Verification items for the finished model (mm, model axes). Face numbers are marked on the shaded views. Round coordinates to 2 decimals unless told otherwise and drop trailing zeros. Write each loop counter-clockwise with the first axis right and the second up, starting at its lowest first coordinate (ties: lowest second). Pieces come first, ordered by that corner, then holes.
from build123d import *

# Parameters (mm, degrees)
SKETCH_1_W          = 4
SKETCH_1_H          = 12
EXTRUDE_1_DEPTH     = 13
SKETCH_2_R          = 1.25
EXTRUDE_2_DEPTH     = 5
SKETCH_3_R          = 1
CUT_EXTRUDE_1_DEPTH = 22.771541057


with BuildPart() as part:
    # 草图1 → 凸台-拉伸1 (new body)
    with BuildSketch(Plane.XY):
        with Locations((2, 6)):
            Rectangle(SKETCH_1_W, SKETCH_1_H)
    extrude(amount=EXTRUDE_1_DEPTH)

    # 草图2 → 凸台-拉伸2 (add)
    with BuildSketch(Plane(origin=(0, 12, 0), x_dir=(1, 0, 0), z_dir=(0, 1, 0))):
        with Locations(Location((2, -5, 0), (0, 0, 270))):
            Circle(SKETCH_2_R)
    extrude(amount=EXTRUDE_2_DEPTH)

    # 草图3 → 切除-拉伸1 (cut, through all)
    with BuildSketch(Plane.XY.offset(13)):
        with Locations((2, 3.59)):
            Circle(SKETCH_3_R)
    extrude(amount=-CUT_EXTRUDE_1_DEPTH, mode=Mode.SUBTRACT)


solid = part.part
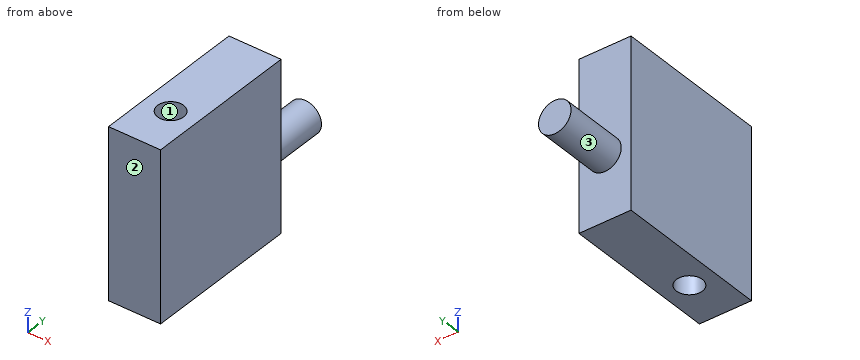
Q1. Depth check by flat-ended pin: P1, Ø1.5, axis at x = 3.5, y = 9, coming from the -Z side; P2, Ø2, axis at x = 2.5, z = 1.5, coming from the +Y side. Enter the tip coordinate at first touch or a pass-through.
Recorded:
P1: stops at z = 0
P2: stops at y = 12
Q2. Sectioned sample at C-C (z = 5). Enter the section's corners in (x, y).
Recorded:
outline: (0, 0) - (4, 0) - (4, 12) - (3.25, 12) - (3.25, 17) - (0.75, 17) - (0.75, 12) - (0, 12) - close; hole circle Ø2 at (2, 3.59)
Q3. Material ranges on line 1 along Y through (x, z) = (2.1, 4.75); line 2 along Y through (x, z) = (2, 9); line 3 along Y through (x, z) = (3.65, 4), recorded low to high.
Recorded:
line 1: y = 0 to 2.6, 4.58 to 17
line 2: y = 0 to 2.59, 4.59 to 12
line 3: y = 0 to 12
Q4. Release check for a two-part mould opening along X. For the marked faces 1, 2 and 3 record: released by +X, released by -X, zero draft, split by the parting line, or undercut.
Recorded:
face 1: undercut
face 2: zero draft
face 3: split by the parting line
Q5. Sectioned sample at B-B (x = 2). Enter the section's corners in (y, z).
Recorded:
outline: (0, 0) - (2.59, 0) - (2.59, 13) - (0, 13) - close; (4.59, 0) - (12, 0) - (12, 3.75) - (17, 3.75) - (17, 6.25) - (12, 6.25) - (12, 13) - (4.59, 13) - close
Q6. Sectioned sample at D-D (z = 11.5). Enter the section's corners in (x, y), plus the area to 3 significant figures.
Recorded:
outline: (0, 0) - (4, 0) - (4, 12) - (0, 12) - close; hole circle Ø2 at (2, 3.59)
area: 44.9 mm2
Q7. Sectioned sample at A-A (y = 3.59). Enter the section's corners in (x, z), plus the area to 3 significant figures.
Recorded:
outline: (0, 0) - (1, 0) - (1, 13) - (0, 13) - close; (3, 0) - (4, 0) - (4, 13) - (3, 13) - close
area: 26.0 mm2
